CAD build for the part. Positions are in the model's coordinates, mm. A direction names the side the tool comes from. Round coordinates to 2 decimals unless told otherwise and drop trailing zeros. Write each loop counter-clockwise with the first axis right and the second up, starting at its lowest first coordinate (ties: lowest second). Pieces come first, ordered by that corner, then holes. Notation, with made-up numbers: (4.25, 17.5) - (29.25, 17.5) arc R27 cw to (29.25, 33.5) - close; hole circle Ø10 at (82, 74.5). An arc over 180 degrees is marked (long way). Put each result on its own line as item: value. Start each with the question number.
Item 1: Pin check, flat tips, straight feed: pin 1 Ø0.5 at (x, y) = (4, 2) entering from +Z; pin 2 Ø0.6 at (x, y) = (-3.5, 1.5) entering from +Z; pin 3 Ø1.5 at (y, z) = (2, 1) entering from +X; pin 4 Ø3 at (x, z) = (0, 0) entering from +Y. Stop position of each tip, or through.
Item 2: Drill centre lines: line 1 (Z direction, x = 0, y = 2.25); line 2 (Z direction, x = 0.25, y = 0.65); line 3 (X direction, y = 2.15, z = 0). Where is each one in solid material? Low to high. Write a range as from..to.
Item 3: 3-axis set-ups, long thin cutter, end or side, ignore diameter. For faces 4 (the flat face through (4, 2, 9.494)), 5 (the flat face through (2.344, 1.521, -7.816)), 6 (the cylindrical face through (-4.72, 1.52, -17.23)), 7 (the cylindrical face through (4.699, 1.521, -17.215)), 8 (the flat face through (-4, 2, 9.494)): which of +Z, -Z, +X, -X, +Y, -Y reach the whole face in a straight line?
Item 4: Mould opens along Z. For faces 1 (the flat face through (0, 1, -17.5)), 2 (the flat face through (-4, 2, 6.494)), 3 (the flat face through (5, 1, 0)) say: released by +Z, released by -Z, zero draft, split by the parting line, or undercut.
Item 5: Cut at A-A (z = 0). Give the cut face in (x, y), and give its area (3 significant figures).
```python
from build123d import *

# Parameters (mm, degrees)
BOSS_EXTRUDE1_OUTLINE_R = 1.783761197
BOSS_EXTRUDE1_DEPTH     = 3
CUT_EXTRUDE1_REACH      = 37.306
FILLET1_R               = 1
FILLET2_R               = 0.5


# Read off the part's stored shape, not the designer's step: Boss-Extrude1
with BuildPart() as part:
    # Boss-Extrude1 outline → Boss-Extrude1 (new body)
    with BuildSketch(Plane(origin=(0, 0, 0), x_dir=(1, 0, 0), z_dir=(0, 1, 0))):
        with BuildLine():
            Line((5, 17.5), (-5, 17.5))
            Line((-5, 17.5), (-6.648887471, -24.389894135))
            add(Edge.make_bspline(
                [(-6.648887471, -24.389894135), (-1.79761276, -31.734966706), (13.203728073, -30.957119403), (24.864765464, -19.062433132), (22.884297555, -6.902852925), (17.013261533, -6.902852925)],
                knots=[0, 0, 0, 0, 0, 0, 1, 1, 1, 1, 1, 1], degree=5))
            add(Edge.make_bspline(
                [(17.013261533, -6.902852925), (17.013261533, -12.122390468), (10.158000359, -21.42084271), (-0.482101901, -21.901454261)],
                knots=[0, 0, 0, 0, 1, 1, 1, 1], degree=3))
            add(Edge.make_bspline(
                [(-0.482101901, -21.901454261), (-2.603887856, -18.477971621), (-1.981580223, -16.222106451), (5, -14.821914277)],
                knots=[0, 0, 0, 0, 1, 1, 1, 1], degree=3))
            Line((5, -14.821914277), (5, 17.5))
        make_face()
        Circle(BOSS_EXTRUDE1_OUTLINE_R, mode=Mode.SUBTRACT)
    extrude(amount=BOSS_EXTRUDE1_DEPTH)

    # Sketch2 → Cut-Extrude1 (cut, up to next)
    with BuildSketch(Plane(origin=(0, 3, 0), x_dir=(1, 0, 0), z_dir=(0, 1, 0)), mode=Mode.PRIVATE) as cut_extrude1_sk1:
        Polygon((-5.438617253, 6.356953165), (-2.423349926, 6.356953165), (-2.259422797, 9.356953165), (-5.320530003, 9.356953165), align=None)
    cut_extrude1_tool1 = extrude(cut_extrude1_sk1.sketch, amount=-CUT_EXTRUDE1_REACH, mode=Mode.PRIVATE) & part.part
    # Sketch2 → Cut-Extrude1 (cut, up to next)
    with BuildSketch(Plane(origin=(0, 3, 0), x_dir=(1, 0, 0), z_dir=(0, 1, 0)), mode=Mode.PRIVATE) as cut_extrude1_sk2:
        Polygon((5, 6.356953165), (2.423349926, 6.356953165), (2.259422797, 9.356953165), (5, 9.356953165), align=None)
    cut_extrude1_tool2 = extrude(cut_extrude1_sk2.sketch, amount=-CUT_EXTRUDE1_REACH, mode=Mode.PRIVATE) & part.part
    # Sketch2 → Cut-Extrude1 (cut, up to next)
    with BuildSketch(Plane(origin=(0, 3, 0), x_dir=(1, 0, 0), z_dir=(0, 1, 0)), mode=Mode.PRIVATE) as cut_extrude1_sk3:
        Polygon((-5.944453926, -6.493799271), (-2.41587233, -6.493799271), (-2.2519452, -9.493799271), (-6.062541177, -9.493799271), align=None)
    cut_extrude1_tool3 = extrude(cut_extrude1_sk3.sketch, amount=-CUT_EXTRUDE1_REACH, mode=Mode.PRIVATE) & part.part
    # Sketch2 → Cut-Extrude1 (cut, up to next)
    with BuildSketch(Plane(origin=(0, 3, 0), x_dir=(1, 0, 0), z_dir=(0, 1, 0)), mode=Mode.PRIVATE) as cut_extrude1_sk4:
        Polygon((5, -6.493799271), (2.41587233, -6.493799271), (2.2519452, -9.493799271), (5, -9.493799271), align=None)
    cut_extrude1_tool4 = extrude(cut_extrude1_sk4.sketch, amount=-CUT_EXTRUDE1_REACH, mode=Mode.PRIVATE) & part.part
    add(cut_extrude1_tool1.solids().sort_by_distance((-3.860303, 3, -7.860725))[0], mode=Mode.SUBTRACT)
    add(cut_extrude1_tool2.solids().sort_by_distance((3.670272, 3, -7.872368))[0], mode=Mode.SUBTRACT)
    add(cut_extrude1_tool3.solids().sort_by_distance((-4.168556, 3, 8.013012))[0], mode=Mode.SUBTRACT)
    add(cut_extrude1_tool4.solids().sort_by_distance((3.666534, 3, 8.009171))[0], mode=Mode.SUBTRACT)

    # Fillet1
    fillet1_edges = [part.edges().sort_by_distance(p)[0] for p in [
        (-5, 1.5, -17.5),
        (5, 1.5, -17.5),
        (5, 1.5, 14.821914277),
        (-6.648887471, 1.5, 24.389894135),
        (17.013261533, 1.5, 6.902852925),
        (-0.482101901, 1.5, 21.901454261),
    ]]
    fillet(fillet1_edges, radius=FILLET1_R)

    # Fillet2
    fillet2_edges = [part.edges().sort_by_distance(p)[0] for p in [
        (5, 1.5, -9.356953165),
        (5, 1.5, -6.356953165),
        (2.423349926, 1.5, -6.356953165),
        (2.259422797, 1.5, -9.356953165),
        (-6.062541177, 1.5, 9.493799271),
        (-5.944453926, 1.5, 6.493799271),
        (-2.41587233, 1.5, 6.493799271),
        (-2.2519452, 1.5, 9.493799271),
        (5, 1.5, 6.493799271),
        (5, 1.5, 9.493799271),
        (2.2519452, 1.5, 9.493799271),
        (2.41587233, 1.5, 6.493799271),
        (-5.438617253, 1.5, -6.356953165),
        (-5.320530003, 1.5, -9.356953165),
        (-2.259422797, 1.5, -9.356953165),
        (-2.423349926, 1.5, -6.356953165),
    ]]
    fillet(fillet2_edges, radius=FILLET2_R)


solid = part.part
```
Output values:
1. pin 1: z = 28.28
1. pin 2: z = 27.29
1. pin 3: x = 5
1. pin 4: through
2. line 1: -17.5..-1.78, 1.78..16.52, 21.86..28.23
2. line 2: -17.5..-1.77, 1.77..16.37, 21.85..28.27
2. line 3: -5.69..-1.78, 1.78..5
3. face 4: +Y, -Y
3. face 5: +X, +Y, -Y
3. face 6: -Z, -X, +Y, -Y
3. face 7: -Z, +X, +Y, -Y
3. face 8: -X, +Y, -Y
4. face 1: released by -Z
4. face 2: undercut
4. face 3: zero draft
5. outline: (-5.69, 0) - (-1.78, 0) - (-1.78, 3) - (-5.69, 3) - close; (1.78, 0) - (5, 0) - (5, 3) - (1.78, 3) - close
5. area: 21.4 mm2
